Model file for the job. Use its own axes, mm. A direction names the side the tool comes from. Coordinates: 2 decimals unless noted, no trailing zeros. Write each loop counter-clockwise with the first axis right and the second up, starting at its lowest first coordinate (ties: lowest second). Pieces come first, ordered by that corner, then holes. Notation, with made-up numbers: M -5,55 L 26,55 A24 cw 26,82 Z; hole C 29,35.5 d2. An arc over 180 degrees is marked long. Answer in a Markdown table with one row per item. Add a question column.
```python
from build123d import *

# Parameters (mm, degrees)
SKETCH1_W           = 71
SKETCH1_H           = 57
BOSS_EXTRUDE1_DEPTH = 3
SKETCH2_W           = 71
SKETCH2_H           = 57
SKETCH2_W_2         = 65
SKETCH2_H_2         = 51
BOSS_EXTRUDE2_DEPTH = 8
SKETCH6_W           = 68
SKETCH6_H           = 54
SKETCH6_W_2         = 65
SKETCH6_H_2         = 51
BOSS_EXTRUDE5_DEPTH = 2
SKETCH7_W           = 26
SKETCH7_H           = 15.829787861
CUT_EXTRUDE2_DEPTH  = 58
SKETCH8_W           = 44
SKETCH8_H           = 23
CUT_EXTRUDE3_DEPTH  = 14
FILLET1_R           = 3


with BuildPart() as part:
    # Sketch1 → Boss-Extrude1 (new body)
    with BuildSketch(Plane(origin=(0, 0, 0), x_dir=(1, 0, 0), z_dir=(0, 1, 0))):
        Rectangle(SKETCH1_W, SKETCH1_H)
    extrude(amount=BOSS_EXTRUDE1_DEPTH)

    # Sketch2 → Boss-Extrude2 (add)
    with BuildSketch(Plane(origin=(0, 3, 0), x_dir=(1, 0, 0), z_dir=(0, 1, 0))):
        Rectangle(SKETCH2_W, SKETCH2_H)
        Rectangle(SKETCH2_W_2, SKETCH2_H_2, mode=Mode.SUBTRACT)
    extrude(amount=BOSS_EXTRUDE2_DEPTH)

    # Sketch6 → Boss-Extrude5 (add)
    with BuildSketch(Plane(origin=(0, 11, 0), x_dir=(1, 0, 0), z_dir=(0, 1, 0))):
        Rectangle(SKETCH6_W, SKETCH6_H)
        Rectangle(SKETCH6_W_2, SKETCH6_H_2, mode=Mode.SUBTRACT)
    extrude(amount=BOSS_EXTRUDE5_DEPTH)

    # Sketch7 → Cut-Extrude2 (cut, through all)
    with BuildSketch(Plane(origin=(0, 0, -28.5), x_dir=(-1, 0, 0), z_dir=(0, 0, -1))):
        with Locations((-22.5, 7.063052876)):
            Rectangle(SKETCH7_W, SKETCH7_H)
    extrude(amount=-CUT_EXTRUDE2_DEPTH, mode=Mode.SUBTRACT)

    # Sketch8 → Cut-Extrude3 (cut, through all)
    with BuildSketch(Plane.XZ):
        with Locations((13.5, 17)):
            Rectangle(SKETCH8_W, SKETCH8_H)
    extrude(amount=-CUT_EXTRUDE3_DEPTH, mode=Mode.SUBTRACT)

    # Fillet1
    fillet1_edges = [part.edges().sort_by_distance(p)[0] for p in [
        (-8.5, 1.5, 5.5),
        (9.5, 1.5, 5.5),
    ]]
    fillet(fillet1_edges, radius=FILLET1_R)


solid = part.part
```
1) Two-plate mould, pull along Z, no slides. Class faces 4 (the face through (8.64, 1.48, 4.6)), 5 (the face through (-32.5, 8, 0)), 6 (the face through (-18, 0, -7)): released by +Z, released by -Z, zero draft, split by the parting line, or undercut.
2) Drill centre lines: probe 1 along Z at (x, y) = (-18, 4.75); probe 2 along Z at (x, y) = (-4, 1); probe 3 along X at (y, z) = (4, 17). Where is each one in solid material? Low to high.
3) Flat gauge pins, fed straight in: pin 1 Ø1 at (y, z) = (12, -7) entering from -X; pin 2 Ø1 at (x, y) = (-18.5, 12) entering from +Z; pin 3 Ø1.5 at (x, y) = (-4.5, 4.5) entering from +Z; pin 4 Ø12 at (x, z) = (-25, -17) entering from -Y. Where does each tip first touch, or does it go through?
4) Which spindle directions (+Z, -Z, +X, -X, +Y, -Y) get a long thin tool onto all of the face, cutting with end or side? Do faces 1 (the face through (-12, 8, -25.5)), 2 (the face through (-34, 12, 0)), 3 (the face through (0, 1, 5.5)). Say none if no direction does.
5) Slice it at A-A (x = -28). Give the cut face in (y, z).
6) Slice it at C-C (y = 6.25). Give the cut face in (x, z), then the cut area to 3 significant figures.
7) Slice it at B-B (z = -2). Give the cut face in (x, y), then the cut area to 3 significant figures.
Ans:
| question | item | result |
|---|---|---|
| 1 | face 4 | released by +Z |
| 1 | face 5 | undercut |
| 1 | face 6 | zero draft |
| 2 | probe 1 | z = -28.5 to -25.5, 25.5 to 28.5 |
| 2 | probe 2 | z = -28.5 to 5.5 |
| 2 | probe 3 | x = -35.5 to -32.5 |
| 3 | pin 1 | stops at x = -34 |
| 3 | pin 2 | stops at z = 27 |
| 3 | pin 3 | stops at z = -25.5 |
| 3 | pin 4 | stops at y = 0 |
| 4 | face 1 | +X, +Y |
| 4 | face 2 | +Z, -Z, -X, +Y |
| 4 | face 3 | +Z, +X, +Y, -Y |
| 5 | outline | M 0,-28.5 L 11,-28.5 L 11,-27 L 13,-27 L 13,-25.5 L 3,-25.5 L 3,25.5 L 13,25.5 L 13,27 L 11,27 L 11,28.5 L 0,28.5 Z |
| 6 | outline | M -35.5,-28.5 L 9.5,-28.5 L 9.5,-25.5 L -32.5,-25.5 L -32.5,25.5 L -8.5,25.5 L -8.5,28.5 L -35.5,28.5 Z |
| 6 | area | 369 mm2 |
| 7 | outline | M -35.5,0 L 9.5,0 L 9.5,3 L -32.5,3 L -32.5,13 L -34,13 L -34,11 L -35.5,11 Z |
| 7 | area | 162 mm2 |
